Geometry check sheet. Reference: the model listing, model coordinates, mm. A direction names the side the tool comes from. Give positions to 0.01 mm unless a question says otherwise; leave off trailing zeros. Write each loop counter-clockwise with the first axis right and the second up, starting at its lowest first coordinate (ties: lowest second). Pieces come first, ordered by that corner, then holes. Notation, with made-up numbers: (67, 89.5) - (74, 89.5) arc R32 cw to (74, 117.5) - close; hole circle Ø11 at (34, 33). An arc over 180 degrees is marked (long way). Use a Markdown table: item, result.
```python
from build123d import *

# Parameters (mm, degrees)
CUT_EXTRUDE1_DEPTH = 20
SKETCH3_R          = 1.25
CUT_EXTRUDE2_DEPTH = 17
SKETCH4_R          = 0.502757778
SKETCH4_R_2        = 0.50259211
CUT_EXTRUDE3_DEPTH = 3
SKETCH5_R          = 2.25
CUT_EXTRUDE4_DEPTH = 6
SKETCH6_R          = 4.1
CUT_EXTRUDE5_DEPTH = 26


with BuildPart() as part:
    # Sketch1 → Revolve1 (revolve)
    with BuildSketch(Plane.XY, mode=Mode.PRIVATE) as revolve1_sk:
        Polygon((7.5, 61.86812787), (15.454011649, 61.86812787), (15.454011649, 21.86812787), (38.123522242, 21.86812787), (38.123522242, 6.86812787), (25, 6.86812787), (25, 13.86812787), (9, 13.86812787), (9, 21.86812787), (7.5, 21.86812787), align=None)
    revolve(revolve1_sk.sketch.rotate(Axis((0, 0, 0), (0, 1, 0)), 90), axis=Axis((0, 0, 0), (0, 1, 0)))

    # Sketch2 → Cut-Extrude1 (cut, symmetric)
    with BuildSketch(Plane.XY):
        with BuildLine():
            Line((-0.897403203, 116.981683018), (0.871590836, 116.981683018))
            Line((0.871590836, 116.981683018), (0.871590836, 25.953330627))
            ThreePointArc((0.871590836, 25.953330627), (-0.012906183, 23.46812787), (-0.897403203, 25.953330627))
            Line((-0.897403203, 25.953330627), (-0.897403203, 116.981683018))
        make_face()
    extrude(amount=CUT_EXTRUDE1_DEPTH, both=True, mode=Mode.SUBTRACT)

    # Sketch3 → Cut-Extrude2 (cut)
    with BuildSketch(Plane(origin=(20, 0, 0), x_dir=(0, 0, -1), z_dir=(1, 0, 0))):
        with Locations((-13, 56.805856976)):
            Circle(SKETCH3_R)
        with Locations((13, 56.805856976)):
            Circle(SKETCH3_R)
    cut_extrude2 = extrude(amount=-CUT_EXTRUDE2_DEPTH, mode=Mode.SUBTRACT)

    # Sketch4 → Cut-Extrude3 (cut)
    with BuildSketch(Plane(origin=(3, 0, 0), x_dir=(0, 0, -1), z_dir=(1, 0, 0))):
        with Locations((13, 56.805856976)):
            Circle(SKETCH4_R)
        with Locations((-13, 56.805856976)):
            Circle(SKETCH4_R_2)
    cut_extrude3 = extrude(amount=-CUT_EXTRUDE3_DEPTH, mode=Mode.SUBTRACT)

    # Mirror1: Cut-Extrude2, Cut-Extrude3 across plane
    add(cut_extrude2.mirror(Plane(origin=(0, 0, 0), x_dir=(0, 0, 1), z_dir=(1, 0, 0))), mode=Mode.SUBTRACT)
    add(cut_extrude3.mirror(Plane(origin=(0, 0, 0), x_dir=(0, 0, 1), z_dir=(1, 0, 0))), mode=Mode.SUBTRACT)

    # Sketch5 → Cut-Extrude4 (cut)
    with BuildSketch(Plane.XZ.offset(-6.86812787)):
        with Locations(Location((31.825233869, 0, 0), (0, 0, 270))):
            Circle(SKETCH5_R)
        with Locations(Location((0, -31.825233869, 0), (0, 0, 270))):
            Circle(SKETCH5_R)
        with Locations(Location((-31.825233869, 0, 0), (0, 0, 270))):
            Circle(SKETCH5_R)
        with Locations(Location((0, 31.825233869, 0), (0, 0, 270))):
            Circle(SKETCH5_R)
    extrude(amount=-CUT_EXTRUDE4_DEPTH, mode=Mode.SUBTRACT)

    # Sketch6 → Cut-Extrude5 (cut)
    with BuildSketch(Plane.XZ.offset(-12.86812787)):
        with Locations(Location((0, 31.825233869, 0), (0, 0, 270))):
            Circle(SKETCH6_R)
        with Locations(Location((31.825233869, 0, 0), (0, 0, 270))):
            Circle(SKETCH6_R)
        with Locations(Location((0, -31.825233869, 0), (0, 0, 270))):
            Circle(SKETCH6_R)
        with Locations(Location((-31.825233869, 0, 0), (0, 0, 270))):
            Circle(SKETCH6_R)
    extrude(amount=-CUT_EXTRUDE5_DEPTH, mode=Mode.SUBTRACT)


solid = part.part
```
1) Section check D-D on z = 0. Count the separate pieces of the cut face and the enclosed holes in it, then the cut area to 3 significant figures.
Working result:
| item | result |
|---|---|
| separate pieces | 4 |
| enclosed holes | 0 |
| area | 1,080 mm² |
2) Section check C-C on x = 13.5. Record the boundary of the cut face in (y, z).
Working result:
| item | result |
|---|---|
| outline | (6.87, -35.65) - (21.87, -35.65) - (21.87, -7.52) - (61.87, -7.52) - (61.87, 7.52) - (21.87, 7.52) - (21.87, 35.65) - (6.87, 35.65) - (6.87, 21.04) - (13.87, 21.04) - (13.87, -21.04) - (6.87, -21.04) - close |
3) Set-up check for faces 1 (the flat face through (0.872, 44, -11)), 2 (the flat face through (-3, 57, -14)), 3 (the cylindrical face through (5.786, 57.181, 11.808)), 4 (the cylindrical face through (0.18, 17.31, 35.92)): record each of +Z, -Z, +X, -X, +Y, -Y from which the full face is reachable in a straight line by a thin tool's end or side.
Working result:
| item | result |
|---|---|
| face 1 | +Z, -Z, +Y |
| face 2 | -X |
| face 3 | +X |
| face 4 | +Y |
4) Material ranges on L1, parallel to X at y = 26, z = 1; L2, parallel to Z at x = -2.5, y = 14.5; L3, parallel to Y at x = 2.4, z = -13, recorded low to high. Write a range as from..to.
Working result:
| item | result |
|---|---|
| L1 | x = -15.42..-7.43, 7.43..15.42 |
| L2 | z = -38.04..-35.07, -28.58..-8.65, 8.65..28.58, 35.07..38.04 |
| L3 | y = 13.87..56.3, 57.31..61.87 |
5) Depth check by flat-ended pin: P1, Ø6, axis at x = -17, y = 34, coming from the +Z side; P2, Ø2.5, axis at x = -0.01, y = 24.87, coming from the +Z side; P3, Ø1.2, axis at y = 57, z = -12.5, coming from the -X side; P4, Ø1.5, axis at x = -3, y = 51.5, coming from the -Z side. Enter the tip coordinate at first touch or a pass-through.
Working result:
| item | result |
|---|---|
| P1 | stops at z = 6.54 |
| P2 | passes through |
| P3 | stops at x = -3 |
| P4 | stops at z = -15.29 |
6) Mould release check, pull along Y, two halves, no side actions. Record for faces 5 (the cylindrical face through (-5.79, 56.86, -11.75)), 6 (the cylindrical face through (-6.083, 17.924, 6.633)), 7 (the flat face through (-1, 6.868, 26)): pulls with the +Y half, pulls with the -Y half, needs draft (parallel to the pull), parting line crosses it, or undercut.
Working result:
| item | result |
|---|---|
| face 5 | undercut |
| face 6 | needs draft |
| face 7 | pulls with the -Y half |
7) Section check B-B on z = 22.5. Record the boundary of the cut face in (x, y), then the cut area to 3 significant figures.
Working result:
| item | result |
|---|---|
| outline | (-30.78, 6.87) - (-10.9, 6.87) - (-10.9, 13.87) - (10.9, 13.87) - (10.9, 6.87) - (30.78, 6.87) - (30.78, 21.87) - (-30.78, 21.87) - close |
| area | 771 mm² |
